Verification items for the finished model (mm, model axes). A direction names the side the tool comes from. Round coordinates to 2 decimals unless told otherwise and drop trailing zeros. Order: outer loops, then holes, each group sorted by start corner. A loop starts at its lowest first (then second) coordinate and runs counter-clockwise, first axis right, second up. Notation, with made-up numbers: M 56,41.5 L 89,41.5 A10 cw 89,45.5 Z; hole C 7.5,22.25 d11. An arc over 180 degrees is marked long. Write item = value, one per line. Start each with the question number.
from build123d import *

# Parameters (mm, degrees)
SKETCH1_W           = 43
SKETCH1_H           = 18
BOSS_EXTRUDE1_DEPTH = 4
CAVITY2_DEPTH       = 2.3
BOSS_EXTRUDE2_DEPTH = 4


# Read off the part's stored shape, not the designer's step: Cavity2
with BuildPart() as part:
    # Sketch1 → Boss-Extrude1 (new body)
    with BuildSketch(Plane.XY):
        Rectangle(SKETCH1_W, SKETCH1_H)
    extrude(amount=BOSS_EXTRUDE1_DEPTH)

    # Cavity2 outline → Cavity2 (cut)
    with BuildSketch(Plane.XY):
        with BuildLine():
            ThreePointArc((-4.514897629, -4.536044466), (0, -6.4), (4.514897629, -4.536044466))
            Line((4.514897629, -4.536044466), (17, -2.7))
            ThreePointArc((17, -2.7), (19.7, 0), (17, 2.7))
            Line((17, 2.7), (4.514897629, 4.536044466))
            ThreePointArc((4.514897629, 4.536044466), (0, 6.4), (-4.514897629, 4.536044466))
            Line((-4.514897629, 4.536044466), (-17, 2.7))
            ThreePointArc((-17, 2.7), (-19.7, 0), (-17, -2.7))
            Line((-17, -2.7), (-4.514897629, -4.536044466))
        make_face()
    extrude(amount=CAVITY2_DEPTH, mode=Mode.SUBTRACT)

    # Sketch4 → Boss-Extrude2 (add)
    with BuildSketch(Plane.XY.offset(4)):
        with BuildLine():
            ThreePointArc((-56.5, 0), (-57.964466094, 3.535533906), (-61.5, 5))
            Line((-61.5, 5), (-61.5, 2))
            ThreePointArc((-61.5, 2), (-60.085786438, 1.414213562), (-59.5, 0))
            ThreePointArc((-59.5, 0), (-60.085786438, -1.414213562), (-61.5, -2))
            Line((-61.5, -2), (-61.5, -5))
            ThreePointArc((-61.5, -5), (-57.964466094, -3.535533906), (-56.5, 0))
        make_face()
        with BuildLine():
            Line((-61.5, 2), (-61.5, 5))
            ThreePointArc((-61.5, 5), (-66.5, 0), (-61.5, -5))
            Line((-61.5, -5), (-61.5, -2))
            ThreePointArc((-61.5, -2), (-63.5, 0), (-61.5, 2))
        make_face()
        with BuildLine():
            Line((-21.5, -5), (-21.5, 5))
            Line((-21.5, 5), (-61.5, 5))
            ThreePointArc((-61.5, 5), (-57.964466094, 3.535533906), (-56.5, 0))
            ThreePointArc((-56.5, 0), (-57.964466094, -3.535533906), (-61.5, -5))
            Line((-61.5, -5), (-21.5, -5))
        make_face()
    extrude(amount=-BOSS_EXTRUDE2_DEPTH)


solid = part.part
1) Gauge pin test, flat ends, axial feed: P1, Ø2, axis at y = 5, z = 3, coming from the -X side; P2, Ø2, axis at y = -6.5, z = 1.5, coming from the -X side; P3, Ø1, axis at y = 2, z = 1.5, coming from the -X side. Record the tip position at first contact, or that the pin passes through.
2) Cross-section at B-B, the plane y = -1. Enter the section's corners in (x, z), then the cut area to 3 significant figures.
3) Release check for a two-part mould opening along Y. For faces 1 (the flat face through (-21.5, 7, 2)), 2 (the flat face through (-42, -5, 2)), 3 (the cylindrical face through (0.1, 6.4, 1.1)), 4 (the flat face through (0, 0, 2.3)) record: pulls with the +Y half, pulls with the -Y half, needs draft (parallel to the pull), parting line crosses it, or undercut.
4) Cross-section at A-A, the plane z = 3.1. Enter the section's corners in (x, y), then the cut area to 3 significant figures.
5) Cross-section at C-C, the plane x = -60.5. Enter the section's corners in (y, z).
6) Scan lines: probe 1 along Y at (x, z) = (-4, 0.45); probe 2 along X at (y, z) = (6, 2.8); probe 3 along X at (y, z) = (-0.25, 3.2). Record each from-to range of solid material in increasing order.
7) Cross-section at D-D, the plane x = -2.5. Enter the section's corners in (y, z).
8) Access from +Z, -Z, +X, -X, +Y, -Y to the whole of each face (thin tool, end or side, straight path). Record for faces 5 (the flat face through (-21.5, -7, 2)), 6 (the flat face through (-13, 0, 4)), 7 (the cylindrical face through (19.7, -0.1, 1.1)), 8 (the flat face through (-41, 5, 2)).
Geometry results:
q1.P1 = -64.5
q1.P2 = -21.5
q1.P3 = -66.27
q2.outline = M -66.4,0 L -63.23,0 L -63.23,4 L -66.4,4 Z; M -59.77,0 L -19.51,0 L -19.51,2.3 L 19.51,2.3 L 19.51,0 L 21.5,0 L 21.5,4 L -59.77,4 Z
q2.area = 248 mm^2
q3.face_1 = needs draft
q3.face_2 = pulls with the -Y half
q3.face_3 = undercut
q3.face_4 = undercut
q4.outline = M -61.5,-5 L -21.5,-5 L -21.5,-9 L 21.5,-9 L 21.5,9 L -21.5,9 L -21.5,5 L -61.5,5 A5 ccw Z; hole C -61.5,0 d4
q4.area = 1,200 mm^2
q5.outline = M -5,0 L -1.73,0 L -1.73,4 L -5,4 Z; M 1.73,0 L 5,0 L 5,4 L 1.73,4 Z
q6.probe_1 = -9 to -5, 5 to 9
q6.probe_2 = -21.5 to 21.5
q6.probe_3 = -66.49 to -63.48, -59.52 to 21.5
q7.outline = M -9,0 L -5.89,0 L -5.89,2.3 L 5.89,2.3 L 5.89,0 L 9,0 L 9,4 L -9,4 Z
q8.face_5 = +Z, -Z, -X, -Y
q8.face_6 = +Z, +X, -X, +Y, -Y
q8.face_7 = -Z
q8.face_8 = +Z, -Z, -X, +Y
